Can you work these out from the model? Positions are in its coordinate system, mm. A direction names the side the tool comes from. Coordinates: 2 decimals unless noted, no trailing zeros. Order: outer loops, then holes, each group sorted by start corner. A loop starts at its lowest first (then second) coordinate and runs counter-clockwise, first axis right, second up. Notation, with made-up numbers: (70, 67) -> (108, 67) arc R11 ccw to (108, 71) -> close; hole circle Ø9 at (64, 9). An arc over 180 degrees is marked (long way). Answer in a Markdown table with one row per item. Add a question column.
1. Will these pins go through, and if not, where does the flat tip stop? pin 1 (7 mm diameter, centred on y = 17, z = 7, fed in from +X); pin 2 (0.7 mm diameter, centred on x = 48.5, y = 26.5, fed in from +Z); pin 3 (1 mm diameter, centred on x = 73.5, y = 9.5, fed in from +Z); pin 4 (4 mm diameter, centred on x = 28.5, z = 7.5, fed in from +Y).
2. Imagine slicing it at B-B on x = 88.5. Write out the boundary of the cut face in (y, z), plus the area to 3 significant figures.
3. If I drill on line 1 along X through (y, z) = (22.5, 9.75); line 2 along X through (y, z) = (19.5, 14.25); line 3 along Z through (x, y) = (54.5, 21.75), over which ranges is the centre line in solid material (lowest first)? Write a range as [from, to].
4. Imagine slicing it at D-D on z = 6.75. Write out the boundary of the cut face in (x, y), plus the area to 3 significant figures.
5. We'd pull the mould along X, two halves only. Please class faces 1 (the face through (53, 15, 2)), 2 (the face through (105, 6.75, 11)), 3 (the face through (2, 15, 4)): pulls with the +X half, pulls with the -X half, needs draft (parallel to the pull), parting line crosses it, or undercut.
6. On a 3-axis mill with a long thin cutter (end or side, diameter ignored), from which of +Z, -Z, +X, -X, +Y, -Y can I reach the whole of each face in a straight line? I mean faces 4 (the face through (105.25, 15, 4)), 5 (the face through (4, 15, 9)), 6 (the face through (3, 22.75, 11)), 7 (the face through (106.75, 15, 14)). Say none if no direction works.
7. Imagine slicing it at A-A on z = 13.25. Write out the boundary of the cut face in (x, y), plus the area to 3 significant figures.
8. Imagine slicing it at C-C on y = 17.75. Write out the boundary of the cut face in (x, z).
Autodesk Fusion 360 part; units mm, degrees
sketch "Base" plane through (0, 0, 0) normal (0, 0, 1) x (1, 0, 0)
  line L0 (2, 2) -> (105.25, 2)
  line L1 (105.25, 2) -> (105.25, 27.6)
  line L2 (105.25, 27.6) -> (2, 27.6)
  line L3 (2, 27.6) -> (2, 2)
  dimension "d1" = 25.6
  dimension "d2" = 103.25
extrude "Extrude1" add sketch "Base" along normal blind 2
sketch "Rail" plane through (0, 0, 2) normal (0, 0, 1) x (-1, 0, 0)
  line L0 (-2, -27.6) -> (-2, -2)
  line L1 (-2, -2) -> (-105.25, -2)
  line L2 (-105.25, -2) -> (-105.25, -27.6)
  line L3 (-105.25, -27.6) -> (-2, -27.6)
  line L4 (-2, -27.6) -> (-105.25, -27.6)
  line L5 (-105.25, -27.6) -> (-105.25, -25.35)
  line L6 (-105.25, -25.35) -> (-2, -25.35)
  line L7 (-2, -25.35) -> (-2, -27.6)
  line L8 (-2, -2) -> (-105.25, -2)
  line L9 (-105.25, -2) -> (-105.25, -3.88)
  line L10 (-105.25, -3.88) -> (-2, -3.88)
  line L11 (-2, -3.88) -> (-2, -2)
  dimension "d5" = 2.25
  dimension "d6" = 1.88
extrude "Extrude2" add sketch "Rail" along normal blind 3 contours L0 L2 L3 L4 L5 L6 L7 | L0 L1 L2 L8 L9 L10 L11
sketch "Hook (1.5mm -> 2mm)" plane through (0, 0, 2) normal (0, 0, 1) x (-1, 0, 0)
  line L0 (-2, -3.88) -> (-105.25, -3.88)
  line L1 (-105.25, -3.88) -> (-105.25, -25.35)
  line L2 (-105.25, -25.35) -> (-2, -25.35)
  line L3 (-2, -25.35) -> (-2, -3.88)
  line L4 (-2, -22.75) -> (-4, -22.75)
  line L5 (-4, -22.75) -> (-4, -6.75)
  line L6 (-4, -6.75) -> (-2, -6.75)
  line L7 (-2, -6.75) -> (-2, -22.75)
  line L8 (-105.25, -22.75) -> (-103.25, -22.75)
  line L9 (-103.25, -22.75) -> (-103.25, -6.75)
  line L10 (-103.25, -6.75) -> (-105.25, -6.75)
  line L11 (-105.25, -6.75) -> (-105.25, -22.75)
  dimension "d9" = 2.6
  dimension "d10" = 16
  dimension "d11" = 3.07
  dimension "d12" = 2
  dimension "d13" = 2
  dimension "d14" = 16
  dimension "d15" = 2.6
  dimension "d16" = 2.87
extrude "Extrude3" add sketch "Hook (1.5mm -> 2mm)" along normal blind 14.5 contours L3 L4 L5 L6 L7 | L1 L8 L9 L10 L11
sketch "Hook Left" plane through (0, 6.75, 0) normal (0, -1, 0) x (1, 0, 0)
  line L0 (2, 2) -> (4, 2)
  line L1 (4, 2) -> (4, 16.5)
  line L2 (4, 16.5) -> (2, 16.5)
  line L3 (2, 16.5) -> (2, 2)
  line L4 (4, 16.5) -> (0.5, 16.5)
  line L5 (0.5, 16.5) -> (0.5, 11.5)
  line L6 (0.5, 11.5) -> (4, 11.5)
  line L7 (4, 11.5) -> (4, 16.5)
  dimension "d19" = 3.5
  dimension "d20" = 5
sketch "Hook Right" plane through (0, 6.75, 0) normal (0, -1, 0) x (1, 0, 0)
  line L0 (103.25, 2) -> (105.25, 2)
  line L1 (105.25, 2) -> (105.25, 16.5)
  line L2 (105.25, 16.5) -> (103.25, 16.5)
  line L3 (103.25, 16.5) -> (103.25, 2)
  line L4 (103.25, 16.5) -> (106.75, 16.5)
  line L5 (106.75, 16.5) -> (106.75, 11.5)
  line L6 (106.75, 11.5) -> (103.25, 11.5)
  line L7 (103.25, 11.5) -> (103.25, 16.5)
  dimension "d21" = 5
  dimension "d22" = 3.5
extrude "Extrude5" add sketch "Hook Left" sketch "Hook Right" against normal blind 16 contours L3 L4 L5 L6 of sketch 2 contours L1 L4 L5 L6
chamfer "Chamfer1" distance 4 distance2 1.5 1 edges at (0.5, 14.75, 16.5) measured on face at (0.5, 12.0833, 14.8333)
chamfer "Chamfer2" distance 1.5 distance2 4 1 edges at (106.75, 14.75, 16.5) measured on face at (104.4167, 12.0833, 16.5)
extrude "Extrude4" add sketch "Hook Left" sketch "Hook Right" against normal blind 16 contours L3 L4 L5 L6 of sketch 2 contours L1 L4 L5 L6
equation "d19 = 1.5 mm + 2 mm"
equation "d22 = 2 mm + 1.5 mm"
Answers follow:
| question | item | result |
|---|---|---|
| 1 | pin 1 | stops at x = 105.25 |
| 1 | pin 2 | stops at z = 5 |
| 1 | pin 3 | stops at z = 2 |
| 1 | pin 4 | passes through |
| 2 | outline | (2, 0) -> (27.6, 0) -> (27.6, 5) -> (25.35, 5) -> (25.35, 2) -> (3.88, 2) -> (3.88, 5) -> (2, 5) -> close |
| 2 | area | 63.6 mm² |
| 3 | line 1 | x = [2, 4], [103.25, 105.25] |
| 3 | line 2 | x = [0.5, 4], [103.25, 106.75] |
| 3 | line 3 | z = [0, 2] |
| 4 | outline | (2, 6.75) -> (4, 6.75) -> (4, 22.75) -> (2, 22.75) -> close; (103.25, 6.75) -> (105.25, 6.75) -> (105.25, 22.75) -> (103.25, 22.75) -> close |
| 4 | area | 64.0 mm² |
| 5 | face 1 | undercut |
| 5 | face 2 | needs draft |
| 5 | face 3 | pulls with the -X half |
| 6 | face 4 | -Z, +X, +Y, -Y |
| 6 | face 5 | +Z |
| 6 | face 6 | +Z, +X, -X |
| 6 | face 7 | +Z, -Z, +X, +Y, -Y |
| 7 | outline | (0.5, 6.75) -> (4, 6.75) -> (4, 22.75) -> (0.5, 22.75) -> close; (103.25, 6.75) -> (106.75, 6.75) -> (106.75, 22.75) -> (103.25, 22.75) -> close |
| 7 | area | 112 mm² |
| 8 | outline | (0.5, 11.5) -> (2, 11.5) -> (2, 0) -> (105.25, 0) -> (105.25, 11.5) -> (106.75, 11.5) -> (106.75, 16.5) -> (103.25, 16.5) -> (103.25, 2) -> (4, 2) -> (4, 16.5) -> (0.5, 16.5) -> close |
